Source: CAD feature listing. Evaluate the final solid. Frame: model axes, mm. Give positions to 0.01 mm unless a question says otherwise; leave off trailing zeros. Order: outer loops, then holes, each group sorted by start corner. A loop starts at its lowest first (then second) coordinate and runs counter-clockwise, first axis right, second up. Notation, with made-up numbers: (64.25, 52) - (93.25, 52) arc R16 ccw to (93.25, 70) - close; hole circle Ø2 at (13.25, 31). An arc over 180 degrees is marked (long way). Use CSV: the item, a comma, the result in double quotes.
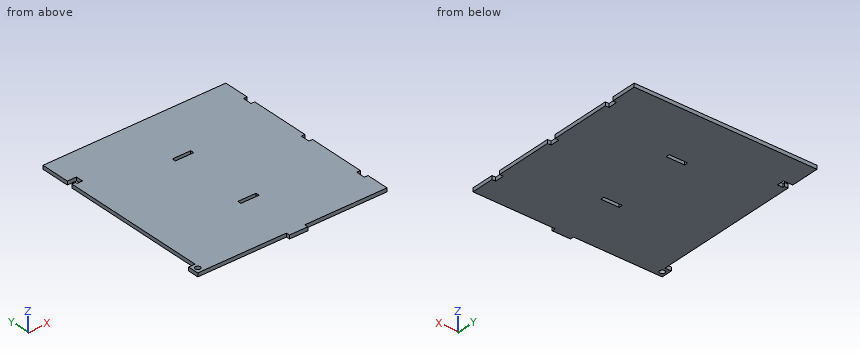
```python
from build123d import *

# Parameters (mm, degrees)
SKETCH1_R           = 1.414213562
SKETCH1_W           = 10
SKETCH1_H           = 2
BOSS_EXTRUDE1_DEPTH = 2


with BuildPart() as part:
    # Sketch1 → Boss-Extrude1 (new body)
    with BuildSketch(Plane.XY):
        Polygon((-53.5, 0), (-50, 0), (-5, 0), (5, 0), (50, 0), (50, 12.5), (48, 12.5), (48, 17.5), (50, 17.5), (50, 30), (50, 49), (48, 49), (48, 54), (50, 54), (50, 73), (50, 87), (48, 87), (48, 92), (50, 92), (50, 106), (-50, 106), (-50, 90), (-45, 90), (-45, 87), (-45, 86), (-48, 86), (-48, 87), (-50, 87), (-50, 6), (-53.5, 6), align=None)
        with Locations((-51, 3)):
            Circle(SKETCH1_R, mode=Mode.SUBTRACT)
        with Locations((0, 31)):
            Rectangle(SKETCH1_W, SKETCH1_H, mode=Mode.SUBTRACT)
        with Locations((0, 74)):
            Rectangle(SKETCH1_W, SKETCH1_H, mode=Mode.SUBTRACT)
        with Locations((0, -1)):
            Rectangle(SKETCH1_W, SKETCH1_H)
    extrude(amount=BOSS_EXTRUDE1_DEPTH)


solid = part.part
```
Item 1: Section D-D on y = 61. Return the cut outline in (x, z), then the cut area to 3 significant figures.
Filled in:
outline,"(-50, 0) - (50, 0) - (50, 2) - (-50, 2) - close"
area,"200 mm2"
Item 2: First-contact query: pin 1 (1 mm diameter, centred on x = 18, z = 1, fed in from -Y); pin 2 (0.6 mm diameter, centred on y = 14.5, z = 1, fed in from +X). Flat tips, straight axial feed; report the tip coordinate or a pass-through.
Filled in:
pin 1,"stops at y = 0"
pin 2,"stops at x = 48"
Item 3: Section A-A on x = 1.5. Return the cut outline in (y, z), then the cut area to 3 significant figures.
Filled in:
outline,"(-2, 0) - (30, 0) - (30, 2) - (-2, 2) - close; (32, 0) - (73, 0) - (73, 2) - (32, 2) - close; (75, 0) - (106, 0) - (106, 2) - (75, 2) - close"
area,"208 mm2"
Item 4: Section C-C on z = 0.95. Count the separate pieces of the cut face and the enclosed holes in it, then the cut area to 3 significant figures.
Filled in:
separate pieces,"1"
enclosed holes,"3"
area,"10,500 mm2"
Item 5: Section B-B on y = 3. Return the cut outline in (x, z).
Filled in:
outline,"(-53.5, 0) - (-52.41, 0) - (-52.41, 2) - (-53.5, 2) - close; (-49.59, 0) - (50, 0) - (50, 2) - (-49.59, 2) - close"
Item 6: Material intervals for line 1 (Y direction, x = -51, z = 0.7); line 2 (X direction, y = 19, z = 0.55); line 3 (Y direction, x = -40, z = 0.9), sorted ascending. Write a range as from..to.
Filled in:
line 1,"y = 0..1.59, 4.41..6"
line 2,"x = -50..50"
line 3,"y = 0..106"
